Drawing for the job (mm, zero at the part's lowest x, y, z). A direction names the side the tool comes from. Coordinates: 2 decimals unless noted, no trailing zeros. Write each loop counter-clockwise with the first axis right and the second up, starting at its lowest first coordinate (ties: lowest second). Pieces come first, ordered by that corner, then holes. Notation, with made-up numbers: (-38, -8) - (-11, -8) arc R24 ccw to (-11, 30) - close; hole circle Ø8 at (4.5, -12.75). An arc over 180 degrees is marked (long way). Write each question's results on one line, items separated by ' | '.
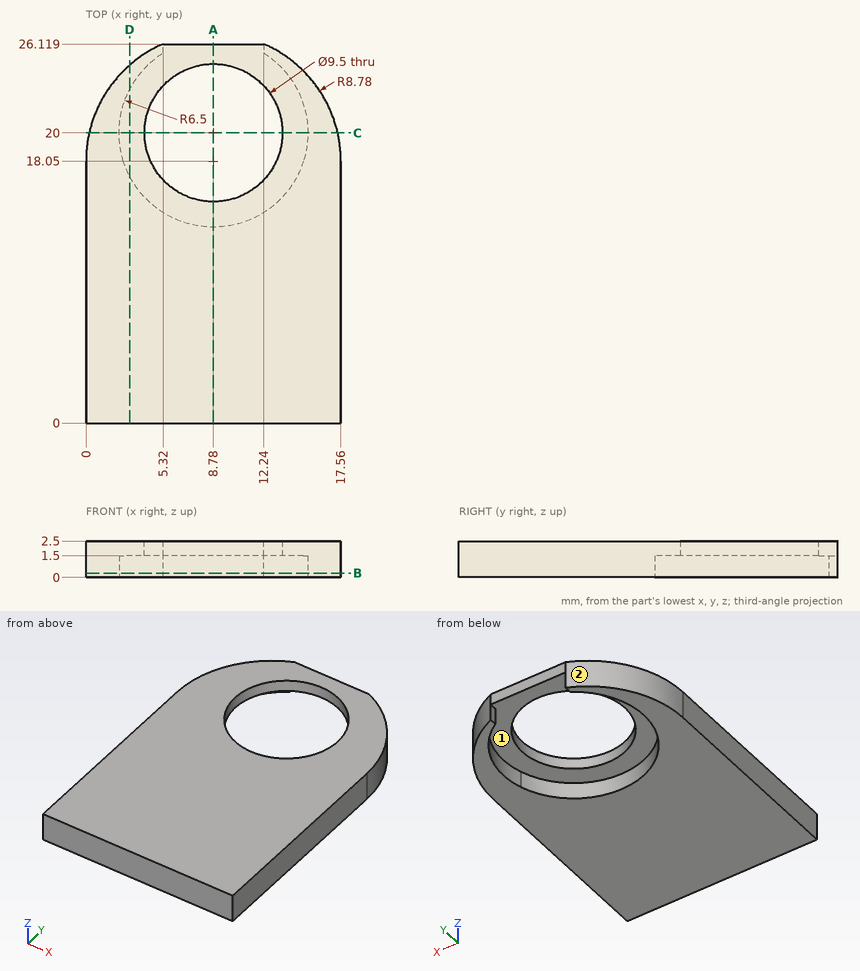
(1) 3-axis set-ups, long thin cutter, end or side, ignore diameter. For the marked faces 1 and 2: which of +Z, -Z, +X, -X, +Y, -Y reach the whole face in a straight line?
Return value:
face 1: -Z | face 2: +Z, -Z, -X, +Y
(2) Flat gauge pin, fed straight in: P1, Ø0.7, axis at y = 25.5, z = 1, coming from the -X side (1 decimal). Where does the tip first touch, or does it go through?
Return value:
P1: stops at x = 3.6
(3) Wall check: line 1 (Y direction, x = 8.78, z = 2.1); line 2 (Z direction, x = 7, y = 14.75); line 3 (Y direction, x = 4.25, z = 0.4). Give the ranges that are in metal, low to high. Write a range as from..to.
Return value:
line 1: y = 0..15.25, 24.75..26.12 | line 2: z = 1.5..2.5 | line 3: y = 0..15.34, 24.66..25.57
(4) Saw through at A-A on x = 8.78. Write the cut outline in (y, z).
Return value:
outline: (0, 0) - (13.5, 0) - (13.5, 1.5) - (15.25, 1.5) - (15.25, 2.5) - (0, 2.5) - close; (24.75, 1.5) - (26.12, 1.5) - (26.12, 2.5) - (24.75, 2.5) - close
(5) Saw through at D-D on x = 3. Write the cut outline in (y, z).
Return value:
outline: (0, 0) - (17.03, 0) - (17.03, 1.5) - (22.97, 1.5) - (22.97, 0) - (24.66, 0) - (24.66, 2.5) - (0, 2.5) - close
(6) Saw through at B-B on z = 0.3. Write the cut outline in (x, y).
Return value:
outline: (0, 0) - (17.56, 0) - (17.56, 18.05) arc R8.78 ccw to (12.24, 26.12) - (12.24, 25.5) arc R6.5 cw (long way) to (5.32, 25.5) - (5.32, 26.12) arc R8.78 ccw to (0, 18.05) - close
(7) Saw through at C-C on y = 20. Write the cut outline in (x, z).
Return value:
outline: (0.22, 0) - (2.28, 0) - (2.28, 1.5) - (4.03, 1.5) - (4.03, 2.5) - (0.22, 2.5) - close; (13.53, 1.5) - (15.28, 1.5) - (15.28, 0) - (17.34, 0) - (17.34, 2.5) - (13.53, 2.5) - close
